Work out the finished part from the listing and answer in its coordinate system (mm). Face numbers are marked on the shaded views. A direction names the side the tool comes from. Give positions to 0.01 mm unless a question says otherwise; leave off trailing zeros. Order: outer loops, then holes, each group sorted by start corner. A loop starts at its lowest first (then second) coordinate and runs counter-clockwise, first axis right, second up.
```python
from build123d import *

# Parameters (mm, degrees)
SKETCH_1_W          = 40
SKETCH_1_H          = 20
EXTRUDE_1_DEPTH     = 39
SKETCH_2_W          = 20
SKETCH_2_H          = 4
EXTRUDE_2_DEPTH     = 7
SKETCH_3_R          = 1.5
CUT_EXTRUDE_1_DEPTH = 4
SKETCH_4_W          = 7
SKETCH_4_H          = 4
EXTRUDE_3_DEPTH     = 20
SKETCH_5_R          = 1.5
CUT_EXTRUDE_2_DEPTH = 4
SKETCH_6_R          = 10
EXTRUDE_4_DEPTH     = 9
SKETCH_7_R          = 1.5
CUT_EXTRUDE_3_DEPTH = 6


with BuildPart() as part:
    # Эскиз1 → Бобышка-Вытянуть1 (new body)
    with BuildSketch(Plane(origin=(0, 0, 0), x_dir=(1, 0, 0), z_dir=(0, 1, 0))):
        Rectangle(SKETCH_1_W, SKETCH_1_H)
    extrude(amount=EXTRUDE_1_DEPTH)

    # Эскиз2 → Бобышка-Вытянуть2 (add)
    with BuildSketch(Plane(origin=(20, 0, 0), x_dir=(0, 0, -1), z_dir=(1, 0, 0))):
        with Locations((0, 29)):
            Rectangle(SKETCH_2_W, SKETCH_2_H)
    extrude(amount=EXTRUDE_2_DEPTH)

    # Эскиз3 → Вырез-Вытянуть1 (cut)
    with BuildSketch(Plane(origin=(0, 31, 0), x_dir=(1, 0, 0), z_dir=(0, 1, 0))):
        with Locations(Location((23.5, 4.5, 0), (0, 0, 270))):
            Circle(SKETCH_3_R)
        with Locations(Location((23.5, -4.5, 0), (0, 0, 270))):
            Circle(SKETCH_3_R)
    extrude(amount=-CUT_EXTRUDE_1_DEPTH, mode=Mode.SUBTRACT)

    # Эскиз4 → Бобышка-Вытянуть3 (add)
    with BuildSketch(Plane.XY.offset(10)):
        with Locations((-23.5, 29)):
            Rectangle(SKETCH_4_W, SKETCH_4_H)
    extrude(amount=-EXTRUDE_3_DEPTH)

    # Эскиз5 → Вырез-Вытянуть2 (cut)
    with BuildSketch(Plane(origin=(0, 31, 0), x_dir=(1, 0, 0), z_dir=(0, 1, 0))):
        with Locations(Location((-23.5, -4.5, 0), (0, 0, 270))):
            Circle(SKETCH_5_R)
        with Locations(Location((-23.5, 4.5, 0), (0, 0, 270))):
            Circle(SKETCH_5_R)
    extrude(amount=-CUT_EXTRUDE_2_DEPTH, mode=Mode.SUBTRACT)

    # Эскиз6 → Бобышка-Вытянуть4 (add)
    with BuildSketch(Plane(origin=(0, 39, 0), x_dir=(1, 0, 0), z_dir=(0, 1, 0))):
        with Locations(Location((10, 0, 0), (0, 0, 270))):
            Circle(SKETCH_6_R)
    extrude(amount=EXTRUDE_4_DEPTH)

    # Эскиз7 → Вырез-Вытянуть3 (cut)
    with BuildSketch(Plane(origin=(0, 48, 0), x_dir=(1, 0, 0), z_dir=(0, 1, 0))):
        with Locations(Location((10, 0, 0), (0, 0, 270))):
            Circle(SKETCH_7_R)
    extrude(amount=-CUT_EXTRUDE_3_DEPTH, mode=Mode.SUBTRACT)


solid = part.part
```
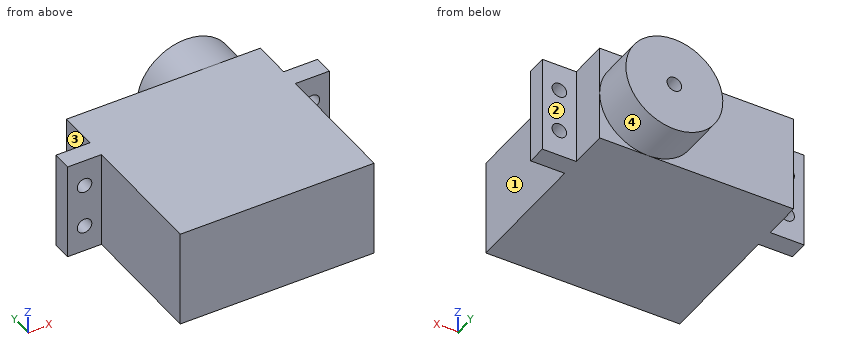
1. The part is cut by section B-B (z = -8). Write down the section's boundary in (x, y).
Findings below:
outline: (-27, 27) - (-20, 27) - (-20, 0) - (20, 0) - (20, 27) - (27, 27) - (27, 31) - (20, 31) - (20, 39) - (16, 39) - (16, 48) - (4, 48) - (4, 39) - (-20, 39) - (-20, 31) - (-27, 31) - close
2. The part is cut by section D-D (y = 23). Write down the section's boundary in (x, z).
Findings below:
outline: (-20, -10) - (20, -10) - (20, 10) - (-20, 10) - close
3. The part is cut by section A-A (x = 23.5). Write down the section's boundary in (y, z), then the cut area to 3 significant figures.
Findings below:
outline: (27, -10) - (31, -10) - (31, -6) - (27, -6) - close; (27, -3) - (31, -3) - (31, 3) - (27, 3) - close; (27, 6) - (31, 6) - (31, 10) - (27, 10) - close
area: 56.0 mm2
4. Given P1, Ø5, axis at y = 38, z = -1, coming from the -X side; P2, Ø3.5, axis at x = 23.5, z = -4.5, coming from the +Y side; P3, Ø4, axis at y = 33.5, z = -2.5, coming from the +X side; P4, Ø2.5, axis at x = -23.5, z = -4.5, coming from the -Y side, each flat-ended and moving along its own axis, determine where each tip first touches the part or whether it passes through.
Findings below:
P1: stops at x = -20
P2: stops at y = 31
P3: stops at x = 20
P4: passes through
5. Which of the six approach directions +Z, -Z, +X, -X, +Y, -Y give full straight-line access (tool end or side, diameter ignored) to the marked faces 1, 2, 3 and 4?
Findings below:
face 1: +Z, -Z, +X, -Y
face 2: +Z, -Z, +X, +Y
face 3: +Z, -Z, -X, +Y
face 4: +Y
6. The part is cut by section C-C (z = 4.5). Write down the section's boundary in (x, y), then the cut area to 3 significant figures.
Findings below:
outline: (-27, 27) - (-25, 27) - (-25, 31) - (-27, 31) - close; (-22, 27) - (-20, 27) - (-20, 0) - (20, 0) - (20, 27) - (22, 27) - (22, 31) - (20, 31) - (20, 39) - (18.93, 39) - (18.93, 48) - (1.07, 48) - (1.07, 39) - (-20, 39) - (-20, 31) - (-22, 31) - close; (25, 27) - (27, 27) - (27, 31) - (25, 31) - close
area: 1,750 mm2
7. Straight lines are drawn through the part: probe 1 along X at (y, z) = (28.95, 4.5); probe 2 along Z at (x, y) = (23, 28); probe 3 along Z at (x, y) = (24.5, 28.5). For each, find the intervals that lie inside material, in ascending order.
Findings below:
probe 1: x = -27 to -25, -22 to 22, 25 to 27
probe 2: z = -10 to -5.91, -3.09 to 3.09, 5.91 to 10
probe 3: z = -10 to -5.62, -3.38 to 3.38, 5.62 to 10
